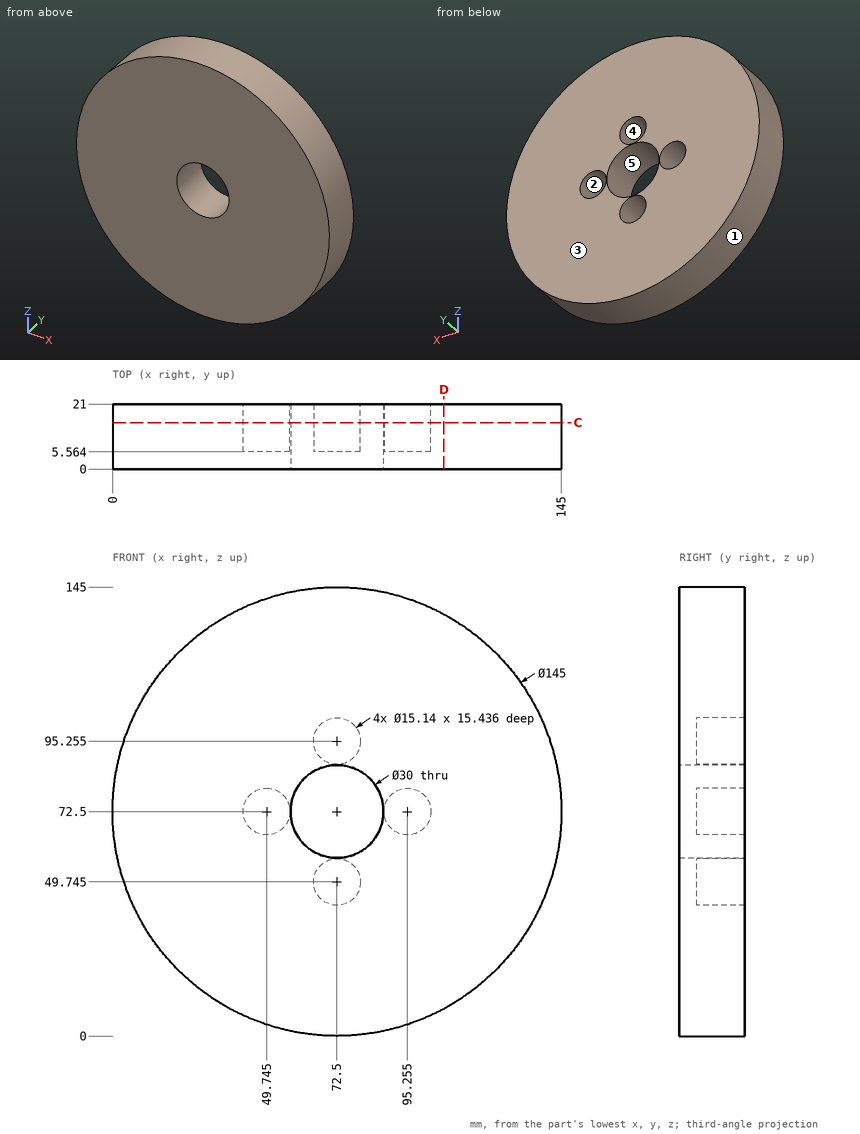
Geometry: see drawing. Coordinates: mm, zero at the bounding-box minimum. A direction names the side the tool comes from. Coordinates: 2 decimals unless noted, no trailing zeros. Write each loop counter-clockwise with the first axis right and the second up, starting at its lowest first coordinate (ties: lowest second). Pieces come first, ordered by that corner, then holes.
1) Section D-D on x = 107. Output: boundary loops of the cut face in (y, z) (1 decimal), and give its area (3 significant figures).
2) Set-up query: the marked faces 4 and 5. Return all of +Z, -Z, +X, -X, +Y, -Y with unobstructed straight access to the full face (end or side cutting, diameter ignored); none if empty.
3) Section C-C on y = 15. Output: boundary loops of the cut face in (x, z) (1 decimal), and give its area (3 significant figures).
4) Material intervals for line 1 along X through (y, z) = (15.25, 72.5) (1 decimal); line 2 along Z through (x, y) = (68, 10.25); line 3 along Z through (x, y) = (69.5, 8.5) (1 decimal), sorted ascending.
5) Mould query, pull axis X, two halves, no side actions, for the marked faces 1, 2 and 3. Classes: pulls with the +X half, pulls with the -X half, needs draft (parallel to the pull), parting line crosses it, or undercut.
6) Pin query (flat end, axial travel): pin 1 Ø2 at (y, z) = (3.5, 40) entering from +X; pin 2 Ø1.5 at (y, z) = (5, 112.5) entering from -X; pin 3 Ø3 at (x, y) = (106, 10.5) entering from -Z (1 decimal). Return the tip coordinate at first contact, or that it passes through.
Check result:
1. outline: (0, 8.7) - (21, 8.7) - (21, 136.3) - (0, 136.3) - close
1. area: 2,680 mm2
2. face 4: +Y
2. face 5: +Y, -Y
3. outline: circle Ø145 at (72.5, 72.5); hole circle Ø15.1 at (49.7, 72.5); hole circle Ø30 at (72.5, 72.5); hole circle Ø15.1 at (72.5, 49.7); hole circle Ø15.1 at (72.5, 95.3); hole circle Ø15.1 at (95.3, 72.5)
3. area: 15,100 mm2
4. line 1: x = 0 to 42.2, 57.3 to 57.5, 87.5 to 87.7, 102.8 to 145
4. line 2: z = 0.14 to 43.66, 55.83 to 58.19, 86.81 to 89.17, 101.34 to 144.86
4. line 3: z = 0.1 to 42.8, 56.7 to 57.8, 87.2 to 88.3, 102.2 to 144.9
5. face 1: parting line crosses it
5. face 2: undercut
5. face 3: needs draft
6. pin 1: stops at x = 137.8
6. pin 2: stops at x = 11.54
6. pin 3: stops at z = 7.4
